CAD build for the part. Positions are in the model's coordinates, mm. Round coordinates to 2 decimals unless told otherwise and drop trailing zeros. Write each loop counter-clockwise with the first axis right and the second up, starting at its lowest first coordinate (ties: lowest second). Pieces come first, ordered by that corner, then holes. Notation, with made-up numbers: (-24.5, 88.25) - (4.5, 88.25) arc R18 cw to (4.5, 112.25) - close; hole circle Ø1 at (24.5, 25.5). An arc over 180 degrees is marked (long way). Answer in a Markdown table with one row per item.
```python
from build123d import *

# Parameters (mm, degrees)
SKETCH1_R           = 1.70053
BOSS_EXTRUDE1_DEPTH = 6.35


with BuildPart() as part:
    # Sketch1 → Boss-Extrude1 (new body)
    with BuildSketch(Plane(origin=(0, 0, 0), x_dir=(1, 0, 0), z_dir=(0, 1, 0))):
        with BuildLine():
            Line((152.4, -78.951070218), (152.4, -95.294257863))
            ThreePointArc((152.4, -95.294257863), (150.97868492, -101.132174142), (147.03287142, -105.663394603))
            ThreePointArc((147.03287142, -105.663394603), (0, -152.4), (-147.03287142, -105.663394603))
            ThreePointArc((-147.03287142, -105.663394603), (-150.97868492, -101.132174142), (-152.4, -95.294257863))
            Line((-152.4, -95.294257863), (-152.4, -78.951070218))
            ThreePointArc((-152.4, -78.951070218), (-145.304042262, -67.554372875), (-131.945714909, -68.893184619))
            ThreePointArc((-131.945714909, -68.893184619), (0, -113.850994317), (131.945714909, -68.893184619))
            ThreePointArc((131.945714909, -68.893184619), (145.304042262, -67.554372875), (152.4, -78.951070218))
        make_face()
        with Locations(Location((117.248460029, -95.925846163, 0), (0, 0, 270))):
            Circle(SKETCH1_R, mode=Mode.SUBTRACT)
        with Locations(Location((137.667738303, -99.066982467, 0), (0, 0, 270))):
            Circle(SKETCH1_R, mode=Mode.SUBTRACT)
        with Locations(Location((75.867733859, -121.822498113, 0), (0, 0, 270))):
            Circle(SKETCH1_R, mode=Mode.SUBTRACT)
        with Locations(Location((64.373888493, -139.521467891, 0), (0, 0, 270))):
            Circle(SKETCH1_R, mode=Mode.SUBTRACT)
        with Locations(Location((-117.248460029, -95.925846163, 0), (0, 0, 90))):
            Circle(SKETCH1_R, mode=Mode.SUBTRACT)
        with Locations(Location((-137.667738303, -99.066982467, 0), (0, 0, 90))):
            Circle(SKETCH1_R, mode=Mode.SUBTRACT)
        with Locations(Location((-64.373888493, -139.521467891, 0), (0, 0, 90))):
            Circle(SKETCH1_R, mode=Mode.SUBTRACT)
        with Locations(Location((-75.867733859, -121.822498113, 0), (0, 0, 90))):
            Circle(SKETCH1_R, mode=Mode.SUBTRACT)
    extrude(amount=BOSS_EXTRUDE1_DEPTH)


solid = part.part
```
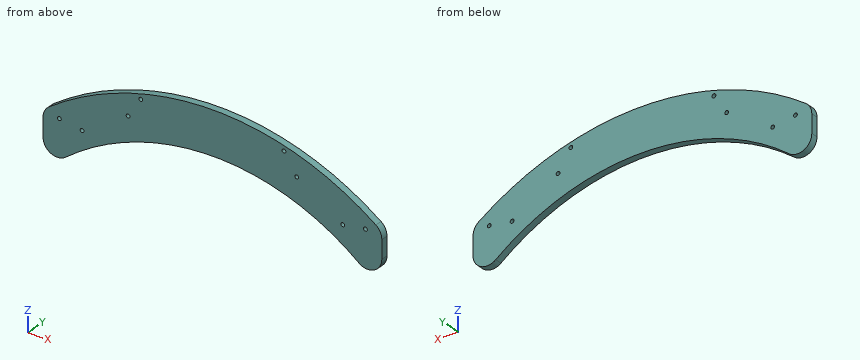
Q1. Flat gauge pins, fed straight in: pin 1 (2 mm diameter, centred on x = -27.5, y = 3.5, fed in from -Z); pin 2 (1.5 mm diameter, centred on y = 5.5, z = 100, fed in from +X). Where does each tip first touch, or does it go through?
Computed:
| item | result |
|---|---|
| pin 1 | stops at z = 111.96 |
| pin 2 | stops at x = 151.77 |
Q2. Saw through at B-B on y = 2. Count the separate pieces of the cut face and the enclosed holes in it, then the cut area to 3 significant figures.
Computed:
| item | result |
|---|---|
| separate pieces | 1 |
| enclosed holes | 8 |
| area | 12,400 mm2 |
Q3. Drill centre lines: line 1 (X direction, y = 0.5, z = 77.5); line 2 (X direction, y = 2.5, z = 81); line 3 (X direction, y = 5.5, z = 125). Where is each one in solid material? Low to high.
Computed:
| item | result |
|---|---|
| line 1 | x = -152.32 to -119.96, 119.96 to 152.32 |
| line 2 | x = -152.4 to -114.54, 114.54 to 152.4 |
| line 3 | x = -114.91 to 114.91 |
Q4. Saw through at D-D on x = -84. List the corners of the cut face in (y, z), then the cut area to 3 significant figures.
Computed:
| item | result |
|---|---|
| outline | (0, 96.86) - (6.35, 96.86) - (6.35, 138.15) - (0, 138.15) - close |
| area | 262 mm2 |
Q5. Saw through at C-C on z = 75. List the corners of the cut face in (x, y), then the cut area to 3 significant figures.
Computed:
| item | result |
|---|---|
| outline | (-151.77, 0) - (-123.62, 0) - (-123.62, 6.35) - (-151.77, 6.35) - close; (123.62, 0) - (151.77, 0) - (151.77, 6.35) - (123.62, 6.35) - close |
| area | 357 mm2 |
Q6. Saw through at A-A on z = 87. List the corners of the cut face in (x, y), then the cut area to 3 significant figures.
Computed:
| item | result |
|---|---|
| outline | (-152.4, 0) - (-104.33, 0) - (-104.33, 6.35) - (-152.4, 6.35) - close; (104.33, 0) - (152.4, 0) - (152.4, 6.35) - (104.33, 6.35) - close |
| area | 611 mm2 |
